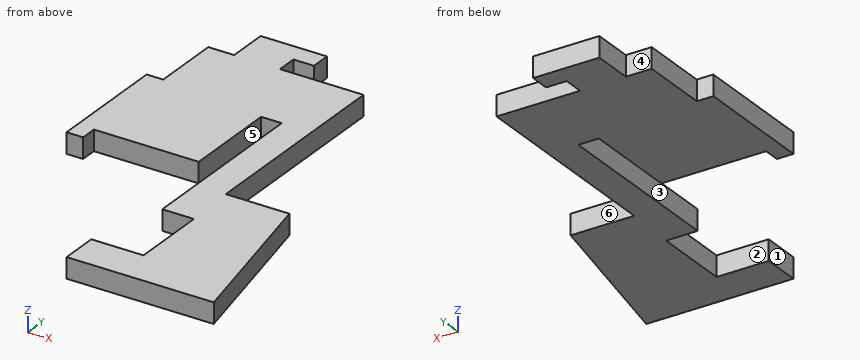
from build123d import *

# Parameters (mm, degrees)
BOSS_EXTRUDE1_DEPTH      = 1.55
BOSS_EXTRUDE1_DEPTH_BACK = 1.55


with BuildPart() as part:
    # Sketch1 → Boss-Extrude1 (new, two sides: drawn at the far end of the back side and taken through both)
    with BuildSketch(Plane.XY.offset(-BOSS_EXTRUDE1_DEPTH_BACK)):
        Polygon((-72.5, 31.1), (-70, 31.1), (-70, 33.6), (-54.19, 33.6), (-54.19, 48), (-51.09, 48), (-51.09, 20.43683659), (-46.319540472, 20.43683659), (-46.319540472, 8.793397686), (-54.19, 8.793397686), (-54.19, 3.1), (-32, 3.1), (-37, 28.21655276), (-46.59, 28.21655276), (-46.59, 60), (-59.19, 60), (-59.19, 63.1), (-56.09, 63.1), (-56.09, 66.1), (-66.09, 66.1), (-66.09, 60), (-70, 60), (-70, 49.6), (-72.5, 49.6), align=None)
    extrude(amount=BOSS_EXTRUDE1_DEPTH + BOSS_EXTRUDE1_DEPTH_BACK)


solid = part.part
Design review of the part built by this model. Coordinates are the model's own, in mm. Face numbers are marked on the shaded views. A direction names the side the tool comes from. Coordinates: 2 decimals unless noted, no trailing zeros. Loops run counter-clockwise (first coordinate to the right, second up) from the corner with the lowest first, then second, coordinate; pieces in that order, holes last. Notation, with made-up numbers: M 72.5,47 L 78.5,47 A15 cw 78.5,58 Z; hole C 31.5,77.25 d11. An arc over 180 degrees is marked long. Use one line per item in the form item = value.
(1) Consider section A-A (y = 46.5). Write out the cut boundary in (x, z), and give its area (3 significant figures).
Return value:
outline = M -72.5,-1.55 L -54.19,-1.55 L -54.19,1.55 L -72.5,1.55 Z; M -51.09,-1.55 L -46.59,-1.55 L -46.59,1.55 L -51.09,1.55 Z
area = 70.7 mm2
(2) For the marked faces 4, 5 and 6, list the 3-axis set-ups (+Z, -Z, +X, -X, +Y, -Y) from which the entire face can be reached by the end or side of a thin tool; tool diameter is ignored.
Return value:
face_4 = +Z, -Z, -X, +Y
face_5 = +Z, -Z
face_6 = +Z, -Z, +X, +Y
(3) Consider section D-D (y = 58.5). Write out the cut boundary in (x, z).
Return value:
outline = M -70,-1.55 L -46.59,-1.55 L -46.59,1.55 L -70,1.55 Z
(4) For line 1 along Y through (x, z) = (-48, 0.9); line 2 along Y through (x, z) = (-56.5, 1.2); line 3 along X through (y, z) = (43.5, -1.3), list the stretches that pass through material, from the lowest coordinate up. Write a range as from..to.
Return value:
line_1 = 3.1..8.79, 20.44..60
line_2 = 33.6..60, 63.1..66.1
line_3 = -72.5..-54.19, -51.09..-46.59
(5) Consider section B-B (x = -48). Write out the cut boundary in (y, z), and give its area (3 significant figures).
Return value:
outline = M 3.1,-1.55 L 8.79,-1.55 L 8.79,1.55 L 3.1,1.55 Z; M 20.44,-1.55 L 60,-1.55 L 60,1.55 L 20.44,1.55 Z
area = 140 mm2
(6) Draft analysis for pull direction X (two halves, no side actions). For the marked faces 1, 2 and 3, state which applies: pulls with the +X half, pulls with the -X half, needs draft (parallel to the pull), parting line crosses it, or undercut.
Return value:
face_1 = pulls with the -X half
face_2 = needs draft
face_3 = undercut
(7) Consider section C-C (z = 1.05). Write out the cut boundary in (x, y), and give its area (3 significant figures).
Return value:
outline = M -72.5,31.1 L -70,31.1 L -70,33.6 L -54.19,33.6 L -54.19,48 L -51.09,48 L -51.09,20.44 L -46.32,20.44 L -46.32,8.79 L -54.19,8.79 L -54.19,3.1 L -32,3.1 L -37,28.22 L -46.59,28.22 L -46.59,60 L -59.19,60 L -59.19,63.1 L -56.09,63.1 L -56.09,66.1 L -66.09,66.1 L -66.09,60 L -70,60 L -70,49.6 L -72.5,49.6 Z
area = 1,070 mm2
(8) Clearance check with flat-ended pins moving along their axes: P1, Ø0.8, axis at x = -71, z = -0.5, coming from the -Y side; P2, Ø1.2, axis at x = -70.5, z = 0, coming from the +Y side. State where each tip first meets the part, or that it passes through.
Return value:
P1 = 31.1
P2 = 60
